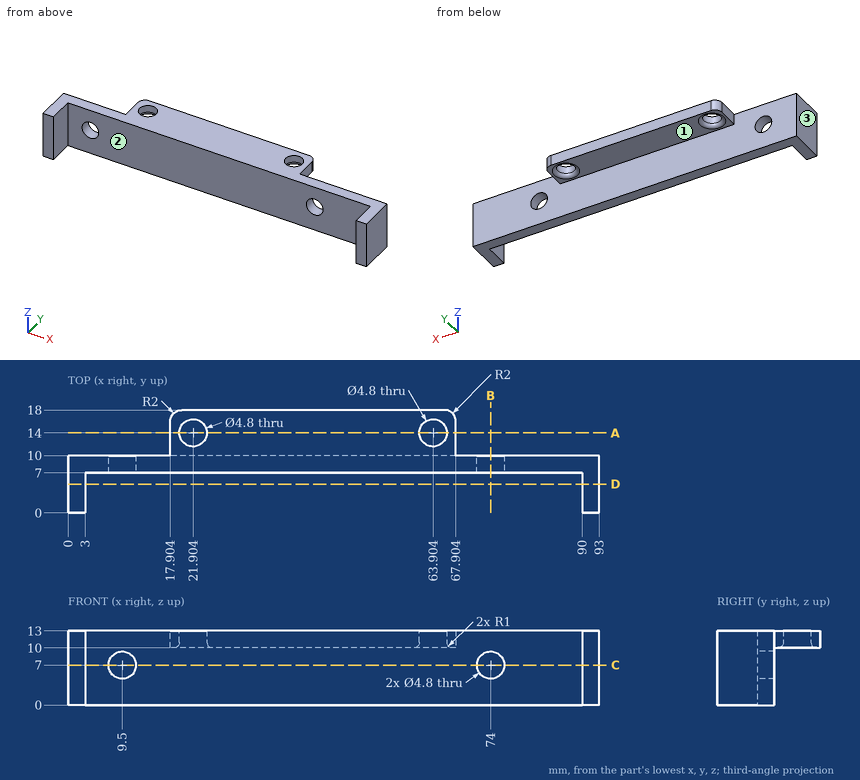
Answer from the drawing. Dimensions are ordinates in mm from the lowest x, y and z of the part. Coordinates: 2 decimals unless noted, no trailing zeros. Write each loop counter-clockwise with the first axis right and the second up, starting at its lowest first coordinate (ties: lowest second). Pieces come first, ordered by that corner, then holes. Notation, with made-up numbers: (-20, 74.25) - (0, 74.25) arc R8 ccw to (0, 87.25) - close; hole circle Ø10 at (-3.5, -34.5). An arc over 180 degrees is marked (long way). Return JSON: item names as keys, results as strings.
1. The part is cut by section A-A on y = 14. Determine the outline of the cut face in (x, z) (1 decimal).
Final values:
{"outline": "(17.9, 10) - (18.5, 10) arc R1 ccw to (19.5, 11) - (19.5, 13) - (17.9, 13) - close; (24.3, 11) arc R1 ccw to (25.3, 10) - (60.5, 10) arc R1 ccw to (61.5, 11) - (61.5, 13) - (24.3, 13) - close; (66.3, 11) arc R1 ccw to (67.3, 10) - (67.9, 10) - (67.9, 13) - (66.3, 13) - close"}
2. Each of these flat-tipped pins is pushed along its axis until it touches: pin 1 Ø2 at (x, z) = (41.5, 4) entering from +Y; pin 2 Ø4 at (x, z) = (9.5, 7) entering from +Y; pin 3 Ø4 at (x, z) = (66.5, 8) entering from -Y; pin 4 Ø0.9 at (y, z) = (11.5, 11.5) entering from +X (1 decimal). Where does it stop, or does it pass through?
Final values:
{"pin 1": "y = 10", "pin 2": "through", "pin 3": "y = 7", "pin 4": "x = 67.9"}
3. The part is cut by section C-C on z = 7. Determine the outline of the cut face in (x, y).
Final values:
{"outline": "(0, 0) - (3, 0) - (3, 7) - (7.1, 7) - (7.1, 10) - (0, 10) - close; (11.9, 7) - (71.6, 7) - (71.6, 10) - (11.9, 10) - close; (76.4, 7) - (90, 7) - (90, 0) - (93, 0) - (93, 10) - (76.4, 10) - close"}
4. The part is cut by section D-D on y = 5. Determine the outline of the cut face in (x, z).
Final values:
{"outline": "(0, 0) - (3, 0) - (3, 13) - (0, 13) - close; (90, 0) - (93, 0) - (93, 13) - (90, 13) - close"}
5. For a pull along X with two mould halves and no side action, classify the marked faces 1, 2 and 3 as +X half, -X half, draft (parallel to the pull), parting line (faces both ways), or undercut.
Final values:
{"face 1": "draft", "face 2": "undercut", "face 3": "-X half"}
6. The part is cut by section B-B on x = 74. Determine the outline of the cut face in (y, z).
Final values:
{"outline": "(7, 0) - (10, 0) - (10, 4.6) - (7, 4.6) - close; (7, 9.4) - (10, 9.4) - (10, 13) - (7, 13) - close"}
7. Consider line 1 along X through (y, z) = (9, 7.25); line 2 along X through (y, z) = (6, 9.5); line 3 along Z through (x, y) = (9.5, 8.65). Determine where each line is inside the solid, lowest interval first.
Final values:
{"line 1": "0 to 7.11, 11.89 to 71.61, 76.39 to 93", "line 2": "0 to 3, 90 to 93", "line 3": "0 to 4.6, 9.4 to 13"}
